Read the model definition and answer for the solid it produces. Units are mm, in the model's axes. A direction names the side the tool comes from. Round coordinates to 2 decimals unless told otherwise and drop trailing zeros. Order: outer loops, then holes, each group sorted by start corner. A loop starts at its lowest first (then second) coordinate and runs counter-clockwise, first axis right, second up. Notation, with made-up numbers: (35, 16) - (79, 16) arc R20 ccw to (79, 40) - close; hole circle Ø10 at (4, 61). An arc over 180 degrees is marked (long way). One line per question, with ' | ' between items. Start each with the question number.
1) The part is cut by section C-C, the plane z = 18.5. Give the vertices of the cut face in (x, y), plus the area to 3 significant figures.
2) For faces 1 (the flat face through (2, 0, 43)), 2 (the flat face through (4, -6, 39)), 3 (the flat face through (0, 0, 0)), determine the directions among +Z, -Z, +X, -X, +Y, -Y from which every point of the face is accessible in a straight line to the end or side of a thin tool.
3) The part is cut by section A-A, the plane y = 0. Give the vertices of the cut face in (x, z).
4) The part is cut by section B-B, the plane x = 0. Give the vertices of the cut face in (y, z), plus the area to 3 significant figures.
5) The mould has two halves that part along Y. Classify faces 4 (the flat face through (4, -2, 43)), 5 (the flat face through (-2, -8, 4)), 6 (the cylindrical face through (10, 3.2, 2)), 7 (the flat face through (4, 0, 41)): pulls with the +Y half, pulls with the -Y half, needs draft (parallel to the pull), parting line crosses it, or undercut.
6) Flat-ended cylindrical pins translate along their axes: pin 1 (6 mm diameter, centred on x = 1.5, z = 23.5, fed in from +Y); pin 2 (6 mm diameter, centred on x = 8, z = 12, fed in from -Y) (3 decimals); pin 3 (2 mm diameter, centred on y = 0.5, z = 25.5, fed in from -X). Find the tip coordinate at first contact, or state that the pin passes through.
7) Straight lines are drawn through the part: line 1 (Z direction, x = 5.5, y = -1.75); line 2 (Z direction, x = 0.75, y = -9.5); line 3 (X direction, y = 0.25, z = 2). For each, find the intervals that lie inside material, in ascending order. Write a range as from..to.
8) The part is cut by section D-D, the plane x = -7.5. Give the vertices of the cut face in (y, z).
from build123d import *

# Parameters (mm, degrees)
F0_R     = 10.5
F1_DEPTH = 4
F2_R     = 8
F3_DEPTH = 39
F4_W     = 7
F4_H     = 5
F7_DEPTH = 3


with BuildPart() as f1:
    # F0 (on Top) → F1 (new body)
    with BuildSketch(Plane.XY):
        Circle(F0_R)
    extrude(amount=F1_DEPTH)

    # F2 (on Top) → F3 (join)
    with BuildSketch(Plane.XY):
        Circle(F2_R)
    extrude(amount=F3_DEPTH)

    # F4 (on Right) → F5 (revolve)
    with BuildSketch(Plane.YZ):
        with Locations((3.5, 41.5)):
            Rectangle(F4_W, F4_H)
    revolve(axis=Axis((0, 0, 41.5), (0, 0, -1)))

    # F6 (on face) → F7 (cut)
    with BuildSketch(Plane.XY.offset(44)):
        with BuildLine():
            Line((6.7082039325, 2), (2, 2))
            Line((2, 2), (2, -2.0000025367))
            Line((2, -2.0000025367), (6.7082031762, -2.0000025367))
            ThreePointArc((6.7082031762, -2.0000025367), (6.9266666671, -1.0105883847), (7, 0))
            ThreePointArc((7, 0), (6.9266668581, 1.010587075), (6.7082039325, 2))
        make_face()
    extrude(amount=-F7_DEPTH, mode=Mode.SUBTRACT)


solid = f1.part
Values:
1) outline: circle Ø16 at (0, 0) | area: 201 mm^2
2) face 1: +Z, +X | face 2: +Z | face 3: -Z, +X, -X, +Y, -Y
3) outline: (-10.5, 0) - (10.5, 0) - (10.5, 4) - (8, 4) - (8, 39) - (7, 39) - (7, 41) - (2, 41) - (2, 44) - (-7, 44) - (-7, 39) - (-8, 39) - (-8, 4) - (-10.5, 4) - close
4) outline: (-10.5, 0) - (10.5, 0) - (10.5, 4) - (8, 4) - (8, 39) - (7, 39) - (7, 44) - (-7, 44) - (-7, 39) - (-8, 39) - (-8, 4) - (-10.5, 4) - close | area: 714 mm^2
5) face 4: undercut | face 5: needs draft | face 6: parting line crosses it | face 7: undercut
6) pin 1: stops at y = 8 | pin 2: stops at y = -6.245 | pin 3: stops at x = -8
7) line 1: z = 0..41 | line 2: z = 0..4 | line 3: x = -10.5..10.5
8) outline: (-7.35, 0) - (7.35, 0) - (7.35, 4) - (2.78, 4) - (2.78, 39) - (-2.78, 39) - (-2.78, 4) - (-7.35, 4) - close
